Autodesk Inventor part; units mm, degrees
ref_plane "Work Plane1" through (0, 0, -130) normal (0, 0, 1) x (1, 0, 0)
ref_plane "YZ Plane" through (0, 0, 0) normal (1, 0, 0) x (0, 1, 0)
ref_plane "XZ Plane" through (0, 0, 0) normal (0, 1, 0) x (-1, 0, 0)
sketch "Sketch1" plane through (0, 0, 0) normal (0, 1, 0) x (-1, 0, 0)
  line L0 (0, 0) -> (260, 0)
  line L1 (260, 0) -> (260, -260)
  line L2 (260, -260) -> (0, -260)
  line L3 (0, -260) -> (0, 0)
  dimension "d0" = 260
  dimension "d1" = 260
extrude "Extrusion1" add sketch "Sketch1" along normal blind 200
sketch "Sketch2" plane through (0, 200, 0) normal (0, 1, 0) x (1, 0, 0)
  line L0 (-260, 0) -> (0, 0)
  line L1 (0, 0) -> (-20, 0)
  line L2 (-20, 0) -> (-20, 20)
  line L3 (-20, 20) -> (0, 20)
  line L4 (0, 20) -> (0, 0)
  line L5 (-260, 260) -> (-260, 0)
  line L6 (-260, 260) -> (-240, 260)
  line L7 (-240, 260) -> (-240, 240)
  line L8 (-240, 240) -> (-260, 240)
  line L9 (-260, 240) -> (-260, 260)
  line L10 (-240, 240) -> (-20, 240)
  line L11 (-20, 240) -> (-20, 20)
  line L12 (-20, 20) -> (-240, 20)
  line L13 (-240, 20) -> (-240, 240)
  dimension "d4" = 20
  dimension "d5" = 20
  dimension "d6" = 20
  dimension "d7" = 20
sketch "Sketch3" plane through (-260, 0, 0) normal (0, 0, 1) x (1, 0, 0)
  line L0 (260, 200) -> (0, 200)
  line L1 (0, 200) -> (20, 200)
  line L2 (20, 200) -> (20, 180)
  line L3 (20, 180) -> (0, 180)
  line L4 (0, 180) -> (0, 200)
  line L5 (260, 0) -> (240, 0)
  line L6 (240, 0) -> (240, 50)
  line L7 (240, 50) -> (260, 50)
  line L8 (260, 50) -> (260, 0)
  line L9 (20, 180) -> (240, 180)
  line L10 (240, 180) -> (240, 50)
  line L11 (240, 50) -> (20, 50)
  line L12 (20, 50) -> (20, 180)
  dimension "d8" = 20
  dimension "d9" = 20
  dimension "d10" = 20
  dimension "d11" = 50
extrude "Extrusion2" cut sketch "Sketch2" against normal blind 150 contours L12 L13 L10 L11
extrude "Extrusion3" cut sketch "Sketch3" against normal blind 260 contours L9 L10 L11 L12
ref_plane "Work Plane1" through (0, 0, -130) normal (0, 0, 1) x (1, 0, 0)
sketch "Sketch4" plane through (0, 0, 0) normal (1, 0, 0) x (0, 0, -1)
  line L0 (260, 200) -> (0, 200)
  line L1 (0, 200) -> (20, 200)
  line L2 (20, 200) -> (20, 180)
  line L3 (20, 180) -> (0, 180)
  line L4 (0, 180) -> (0, 200)
  line L5 (260, 0) -> (240, 0)
  line L6 (240, 0) -> (240, 50)
  line L7 (240, 50) -> (260, 50)
  line L8 (260, 50) -> (260, 0)
  line L9 (20, 180) -> (240, 180)
  line L10 (240, 180) -> (240, 50)
  line L11 (240, 50) -> (20, 50)
  line L12 (20, 50) -> (20, 180)
  point P0 (0, 0)
  dimension "d17" = 20
  dimension "d18" = 20
  dimension "d19" = 20
  dimension "d20" = 50
extrude "Extrusion4" cut sketch "Sketch4" against normal blind 260 contours L9 L10 L11 L12
sketch "Sketch5" plane through (0, 200, 0) normal (0, 1, 0) x (1, 0, 0)
  line L0 (-260, 0) -> (0, 0)
  line L1 (-260, 260) -> (0, 260)
  line L2 (0, 260) -> (0, 0)
  line L3 (0, 0) -> (-260, 0)
  line L4 (-260, 0) -> (-260, 260)
  line L5 (-260, 260) -> (-210, 260)
  line L6 (-210, 260) -> (-210, 210)
  line L7 (-210, 210) -> (-260, 210)
  line L8 (-260, 210) -> (-260, 260)
  line L9 (0, 0) -> (-50, 0)
  line L10 (-50, 0) -> (-50, 50)
  line L11 (-50, 50) -> (0, 50)
  line L12 (0, 50) -> (0, 0)
  line L13 (-50, 50) -> (-210, 50)
  line L14 (-210, 50) -> (-210, 210)
  line L15 (-210, 210) -> (-50, 210)
  line L16 (-50, 210) -> (-50, 50)
  dimension "d23" = 50
  dimension "d24" = 50
  dimension "d25" = 50
  dimension "d26" = 50
extrude "Extrusion5" add sketch "Sketch5" along normal blind 10 contours L4 L7 L14 L13 L10 L0 | L10 L11 L2 L0 | L4 L1 L6 L7 | L16 L15 L6 L1 L2 L11
sketch "Sketch6" plane through (0, 210, 0) normal (0, 1, 0) x (1, 0, 0)
  line L0 (0, 0) -> (-130, 0)
  line L1 (-130, 0) -> (-130, 130)
  line L2 (-130, 130) -> (0, 130)
  line L3 (0, 130) -> (0, 0)
  circle A0 centre (-130, 130) radius 97.5
  circle A1 centre (-130, 130) radius 111.25
  circle A2 centre (-130, 130) radius 104.375
  circle A3 centre (-25.625, 130) radius 1.25
  dimension "d33" = 208.75
  dimension "d29" = 130
  dimension "d30" = 130
  dimension "d31" = 195
  dimension "d32" = 222.5
  dimension "d43" = 2.5
sketch "Sketch7" plane through (0, 210, 0) normal (0, 1, 0) x (1, 0, 0)
  circle A0 centre (-25.625, 130) radius 2.5
  circle A1 centre (-25.625, 130) radius 5
  point P0 (0, 0)
  dimension "d37" = 10
extrude "Extrusion7" add sketch "Sketch7" along normal blind 5
sketch "Sketch8" plane through (0, 50, 0) normal (0, 1, 0) x (1, 0, 0)
  line L0 (-20, 0) -> (-240, 0)
  line L1 (0, 240) -> (0, 20)
  point P0 (0, 0)
  point P1 (-130, 0)
  point P2 (0, 130)
  point P3 (-130, 130)
extrude "Extrusion8" add sketch "Sketch6" along normal blind 15 contours A3 A2 L2 | L2 A2 A3 | A2 L2 A3 | A3 L2 A2
pattern_circular "Circular Pattern2" count 4 over 360 about axis through (-130, 50, -130) along (0, 1, 0) of "Extrusion8", "Extrusion7"
properties part number "BaseMk1"
Check sheet for the modelled part. Datum: model origin and axes. Units: mm. A direction names the side the tool comes from. Round coordinates to 2 decimals unless told otherwise and drop trailing zeros. Loops run counter-clockwise (first coordinate to the right, second up) from the corner with the lowest first, then second, coordinate; pieces in that order, holes last. Notation, with made-up numbers: (64.25, -33) - (107.25, -33) arc R25 cw to (107.25, 0) - close; hole circle Ø9 at (66.25, -26). An arc over 180 degrees is marked (long way). Answer as a JSON object with one key per item and string values. Group by question number.
Q1. Mould release check, pull along Z, two halves, no side actions. Record for faces 1 (the face through (-23, 215, -128)), 2 (the face through (-10, 180, -128)): released by +Z, released by -Z, zero draft, split by the parting line, or undercut.
Q2. Scan lines: line 1 along Z through (x, y) = (-18, 125); line 2 along Y through (x, z) = (-109.5, -237.5). Record each from-to range of solid material in increasing order. Write a range as [from, to].
Q3. Set-up check for faces 3 (the face through (-229, 200, -132)), 4 (the face through (-237, 215, -132)), 5 (the face through (-240, 114, -250)): record each of +Z, -Z, +X, -X, +Y, -Y from which the full face is reachable in a straight line by a thin tool's end or side.
Q4. Sectioned sample at A-A, the plane z = -79. Enter the section's corners in (x, y), plus the area to 3 significant figures.
Q5. Sectioned sample at C-C, the plane x = -191. Enter the section's corners in (y, z).
Q6. Sectioned sample at B-B, the plane y = 56.5. Enter the section's corners in (x, z), plus the area to 3 significant figures.
Solution:
{
 "1": {"face 1": "zero draft", "face 2": "undercut"},
 "2": {"line 1": "z = [-260, -240], [-20, 0]", "line 2": "y = [0, 50], [200, 210]"},
 "3": {"face 3": "none", "face 4": "+Y", "face 5": "+Z, -Z"},
 "4": {"outline": "(-260, 0) - (0, 0) - (0, 50) - (-260, 50) - close; (-260, 180) - (-240, 180) - (-240, 200) - (-210, 200) - (-210, 210) - (-260, 210) - close; (-50, 200) - (-20, 200) - (-20, 180) - (0, 180) - (0, 210) - (-50, 210) - close", "area": "14,800 mm²"},
 "5": {"outline": "(0, -260) - (50, -260) - (50, 0) - (0, 0) - close; (180, -260) - (210, -260) - (210, -210) - (200, -210) - (200, -240) - (180, -240) - close; (180, -20) - (200, -20) - (200, -50) - (210, -50) - (210, 0) - (180, 0) - close"},
 "6": {"outline": "(-260, -260) - (-240, -260) - (-240, -240) - (-260, -240) - close; (-260, -20) - (-240, -20) - (-240, 0) - (-260, 0) - close; (-20, -260) - (0, -260) - (0, -240) - (-20, -240) - close; (-20, -20) - (0, -20) - (0, 0) - (-20, 0) - close", "area": "1,600 mm²"}
}
